Can you work these out from the drawing? Everything is in mm from the part's minimum corner. A direction names the side the tool comes from. Coordinates: 2 decimals unless noted, no trailing zeros. Order: outer loops, then holes, each group sorted by start corner. A loop starts at its lowest first (then second) coordinate and runs counter-clockwise, first axis right, second up. Notation, with made-up numbers: (48, -14) - (79, -14) arc R29 ccw to (79, 6) - close; hole circle Ø10 at (-32.75, 20). An arc over 180 degrees is marked (long way). One line per item, written item: value.
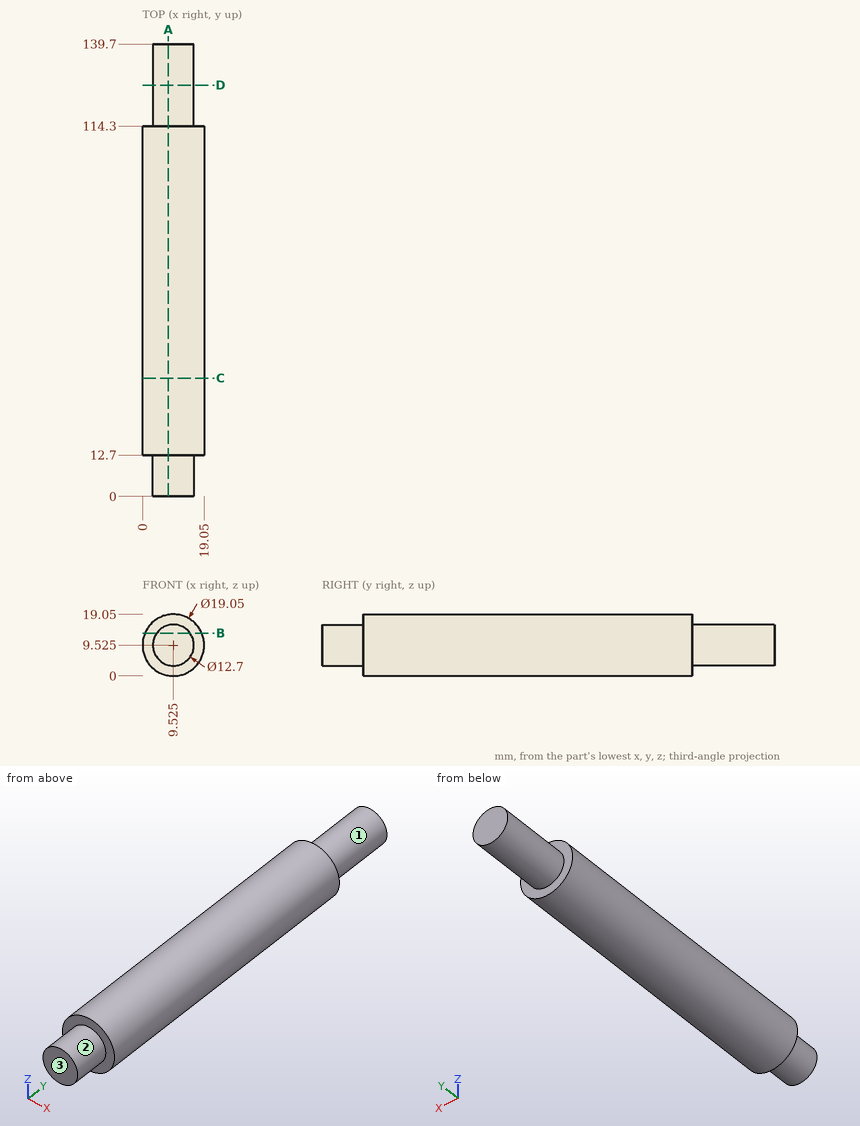
Item 1: I want a section at C-C on y = 36.5. Please give me the cut outline in (x, z) (3 decimals), then the cut area to 3 significant figures.
Conclusion:
outline: circle Ø19.05 at (9.525, 9.525)
area: 285 mm²
Item 2: For the marked faces 1, 2 and 3, which set-ups out of +Z, -Z, +X, -X, +Y, -Y let a thin tool reach every point of the face, with its end or its side?
Conclusion:
face 1: +Y
face 2: -Y
face 3: +Z, -Z, +X, -X, -Y
Item 3: I want a section at D-D on y = 127. Please give me the cut outline in (x, z) (3 decimals), then the cut area to 3 significant figures.
Conclusion:
outline: circle Ø12.7 at (9.525, 9.525)
area: 127 mm²
Item 4: I want a section at B-B on z = 13.25. Please give me the cut outline in (x, y).
Conclusion:
outline: (0.76, 12.7) - (4.38, 12.7) - (4.38, 0) - (14.67, 0) - (14.67, 12.7) - (18.29, 12.7) - (18.29, 114.3) - (14.67, 114.3) - (14.67, 139.7) - (4.38, 139.7) - (4.38, 114.3) - (0.76, 114.3) - close
Item 5: I want a section at A-A on x = 8. Please give me the cut outline in (y, z), then the cut area to 3 significant figures.
Conclusion:
outline: (0, 3.36) - (12.7, 3.36) - (12.7, 0.12) - (114.3, 0.12) - (114.3, 3.36) - (139.7, 3.36) - (139.7, 15.69) - (114.3, 15.69) - (114.3, 18.93) - (12.7, 18.93) - (12.7, 15.69) - (0, 15.69) - close
area: 2,380 mm²
Item 6: I'm going to push flat-ended pins straight in: pin 1 Ø10 at (x, y) = (10, 31.5) entering from -Z; pin 2 Ø1 at (y, z) = (56, 11.5) entering from +X; pin 3 Ø2 at (y, z) = (58, 13) entering from -X; pin 4 Ø1.5 at (y, z) = (78, 16.5) entering from +X. Where does each tip first touch, or does it pass through?
Conclusion:
pin 1: z = 0
pin 2: x = 18.94
pin 3: x = 0.33
pin 4: x = 16.73
Item 7: If I drill on probe 1 along Y at (x, z) = (1, 12.5); probe 2 along X at (y, z) = (49, 10.25); probe 3 along Z at (x, y) = (9.25, 122), over which ranges is the centre line in solid material (lowest first)?
Conclusion:
probe 1: 12.7 to 114.3
probe 2: 0.03 to 19.02
probe 3: 3.18 to 15.87
